Source: CAD feature listing. Evaluate the final solid. Frame: model axes, mm. Face numbers are marked on the shaded views. Round coordinates to 2 decimals unless told otherwise and drop trailing zeros. Order: outer loops, then holes, each group sorted by start corner. A loop starts at its lowest first (then second) coordinate and runs counter-clockwise, first axis right, second up. Notation, with made-up numbers: (59, 77) - (94, 77) arc R14 cw to (94, 85) - close; hole circle Ø3 at (-20.5, 39). An arc over 180 degrees is marked (long way). Return JSON: item names as keys, results as strings. Group by question number.
1) Section C-C, the plane y = 11.25. Return loops of the section in (x, z), plus the area to 3 significant figures.
2) Section B-B, the plane z = 0. Return loops of the section in (x, y).
3) Ray query, line 1 (Z direction, x = 0, y = 9.75); line 2 (X direction, y = 7.75, z = 4.5). Return the intervals inside material, ascending. Write a range as from..to.
4) Section A-A, the plane x = 0. Return loops of the section in (y, z).
5) Contact query for flat-ended pins moving along their axis: P1, Ø5, axis at y = 3.5, z = 6, coming from the +X side; P2, Ø5, axis at x = -6.5, y = 7, coming from the -Z side; P3, Ø5, axis at x = -1, z = -7.5, coming from the +Y side; P4, Ø8.5, axis at x = 0, z = 0, coming from the -Y side. Output: stop coordinate, or through.
6) Mould query, pull axis Z, two halves, no side actions, for the marked faces 1, 2 and 3. Classes: pulls with the +Z half, pulls with the -Z half, needs draft (parallel to the pull), parting line crosses it, or undercut.
```python
from build123d import *


with BuildPart() as part:
    # Sketch1 → Revolve1 (revolve)
    with BuildSketch(Plane.XY):
        with BuildLine():
            Line((3.302, 0), (9.9314, 0))
            ThreePointArc((9.9314, 0), (11.368240979, 0.595159021), (11.9634, 2.032))
            Line((11.9634, 2.032), (11.9634, 12))
            Line((11.9634, 12), (11.1252, 12))
            Line((11.1252, 12), (11.1252, 1.8382))
            ThreePointArc((11.1252, 1.8382), (10.832306781, 1.131093219), (10.1252, 0.8382))
            Line((10.1252, 0.8382), (3.302, 0.8382))
            Line((3.302, 0.8382), (3.302, 0))
        make_face()
    revolve(axis=Axis((0, 0, 0), (0, 1, 0)))


solid = part.part
```
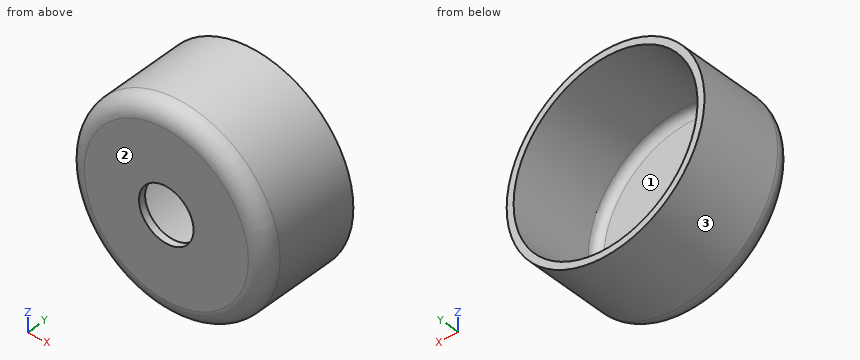
Geometry check:
{
 "1": {"outline": "circle Ø23.93 at (0, 0); hole circle Ø22.25 at (0, 0)", "area": "60.8 mm2"},
 "2": {"outline": "(-11.96, 2.03) arc R2.03 ccw to (-9.93, 0) - (-3.3, 0) - (-3.3, 0.84) - (-10.13, 0.84) arc R1 cw to (-11.13, 1.84) - (-11.13, 12) - (-11.96, 12) - close; (3.3, 0) - (9.93, 0) arc R2.03 ccw to (11.96, 2.03) - (11.96, 12) - (11.13, 12) - (11.13, 1.84) arc R1 cw to (10.13, 0.84) - (3.3, 0.84) - close"},
 "3": {"line 1": "-11.96..-11.13, 11.13..11.96", "line 2": "-11.08..-10.17, 10.17..11.08"},
 "4": {"outline": "(0, -9.93) arc R2.03 ccw to (2.03, -11.96) - (12, -11.96) - (12, -11.13) - (1.84, -11.13) arc R1 cw to (0.84, -10.13) - (0.84, -3.3) - (0, -3.3) - close; (0, 3.3) - (0.84, 3.3) - (0.84, 10.13) arc R1 cw to (1.84, 11.13) - (12, 11.13) - (12, 11.96) - (2.03, 11.96) arc R2.03 ccw to (0, 9.93) - close"},
 "5": {"P1": "x = 11.44", "P2": "z = -11.27", "P3": "y = 0.84", "P4": "y = 0"},
 "6": {"face 1": "undercut", "face 2": "needs draft", "face 3": "parting line crosses it"}
}
